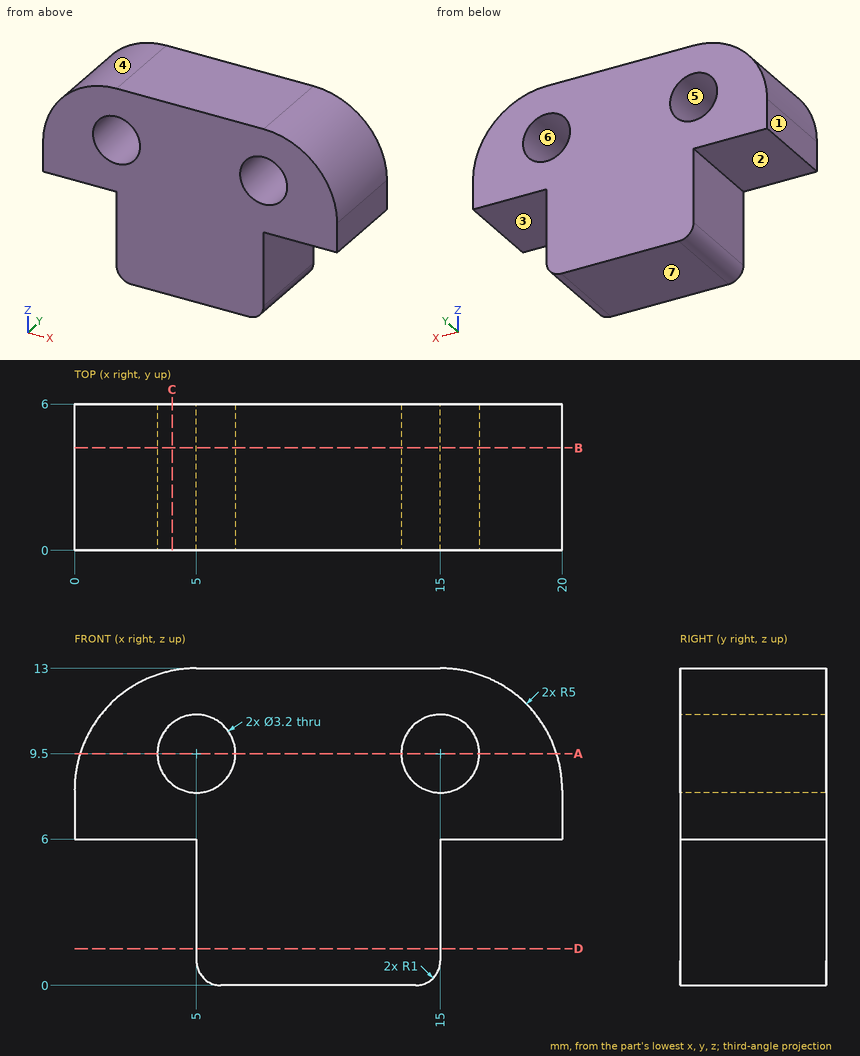
Here's the drawing with two shaded views (mm, measured from the low corner). I have some questions. A direction names the side the tool comes from. Give positions to 0.01 mm unless a question says otherwise; leave off trailing zeros. Write each loop counter-clockwise with the first axis right and the second up, starting at its lowest first coordinate (ties: lowest second). Pieces come first, ordered by that corner, then holes. Notation, with made-up numbers: (49.25, 64.5) - (68.25, 64.5) arc R30 ccw to (68.25, 92.5) - close; hole circle Ø1 at (32, -18.75). An arc over 180 degrees is marked (long way). One line per item, written item: value. Start each with the question number.
Item 1: Imagine slicing it at D-D, the plane z = 1.5. List the corners of the cut face in (x, y) for me, and give its area (3 significant figures).
Item 2: Imagine slicing it at B-B, the plane y = 4.2. List the corners of the cut face in (x, z) for me.
Item 3: Which directions (+Z, -Z, +X, -X, +Y, -Y) give clear straight access to the entire face, cutting with the end or side of a thin tool? Please do the marked faces 1, 2 and 3.
Item 4: Please list where these lines run through material, in increasing order: line 1 (X direction, y = 2.45, z = 9.5); line 2 (X direction, y = 3.4, z = 9.75); line 3 (X direction, y = 2.4, z = 4). Write a range as from..to.
Item 5: If we mould it in two halves opening along X, with no side actions, what happens to the marked faces 4, 5, 6 and 7? For each: +X half, -X half, draft (parallel to the pull), parting line (faces both ways), or undercut.
Item 6: Imagine slicing it at C-C, the plane x = 4. List the corners of the cut face in (y, z) for me.
Item 7: Imagine slicing it at A-A, the plane z = 9.5. List the corners of the cut face in (x, y) for me.
Item 8: I'm going to push flat-ended pins straight in: pin 1 (3.5 mm diameter, centred on x = 15, z = 9.5, fed in from -Y); pin 2 (1.5 mm diameter, centred on x = 18.5, y = 3.5, fed in from -Z); pin 3 (2.5 mm diameter, centred on y = 2.5, z = 4.5, fed in from +X); pin 4 (1.9 mm diameter, centred on x = 5, z = 9.5, fed in from +Y). Where does each tip first touch, or does it pass through?
Geometry says:
1. outline: (5, 0) - (15, 0) - (15, 6) - (5, 6) - close
1. area: 60.0 mm^2
2. outline: (0, 6) - (5, 6) - (5, 1) arc R1 ccw to (6, 0) - (14, 0) arc R1 ccw to (15, 1) - (15, 6) - (20, 6) - (20, 8) arc R5 ccw to (15, 13) - (5, 13) arc R5 ccw to (0, 8) - close; hole circle Ø3.2 at (5, 9.5); hole circle Ø3.2 at (15, 9.5)
3. face 1: +Z, -Z, -X, +Y, -Y
3. face 2: -Z, -X, +Y, -Y
3. face 3: -Z, +X, +Y, -Y
4. line 1: 0.23..3.4, 6.6..13.4, 16.6..19.77
4. line 2: 0.32..3.42, 6.58..13.42, 16.58..19.68
4. line 3: 5..15
5. face 4: -X half
5. face 5: undercut
5. face 6: undercut
5. face 7: draft
6. outline: (0, 6) - (6, 6) - (6, 8.25) - (0, 8.25) - close; (0, 10.75) - (6, 10.75) - (6, 12.9) - (0, 12.9) - close
7. outline: (0.23, 0) - (3.4, 0) - (3.4, 6) - (0.23, 6) - close; (6.6, 0) - (13.4, 0) - (13.4, 6) - (6.6, 6) - close; (16.6, 0) - (19.77, 0) - (19.77, 6) - (16.6, 6) - close
8. pin 1: y = 0
8. pin 2: z = 6
8. pin 3: x = 15
8. pin 4: through
